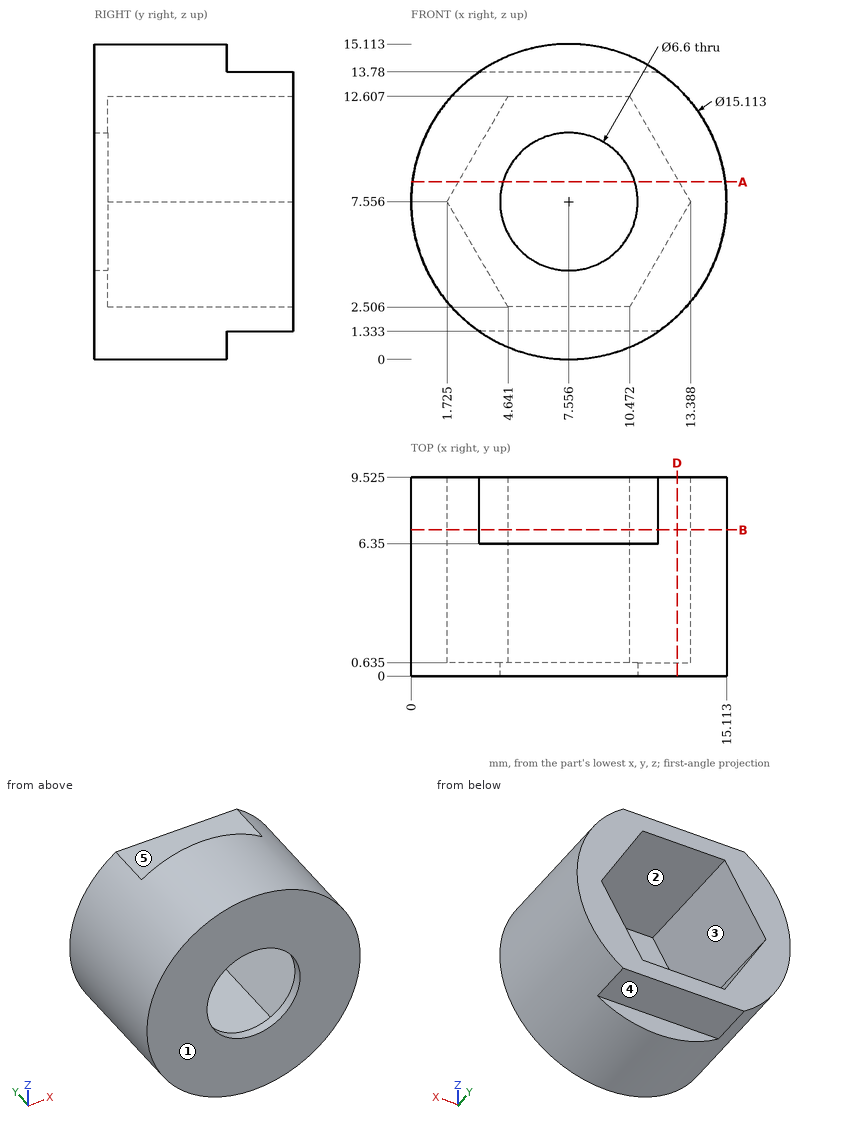
Geometry check sheet. Reference: drawing and pictorial views, mm from the part's lowest x, y, z. A direction names the side the tool comes from. Give positions to 0.01 mm unless a question says otherwise; leave off trailing zeros. Loops run counter-clockwise (first coordinate to the right, second up) from the corner with the lowest first, then second, coordinate; pieces in that order, holes last. Notation, with made-up numbers: (58, 71) -> (73, 71) arc R22 cw to (73, 98) -> close; hole circle Ø6 at (-37.5, 44.25). An arc over 180 degrees is marked (long way). Answer in a Markdown table with one row per item. Add a question column.
1) Material ranges on probe 1 along Z at (x, y) = (8.25, 9.25); probe 2 along Y at (x, z) = (5.5, 11) (1 decimal); probe 3 along Z at (x, y) = (10.5, 8) (1 decimal), recorded low to high. Write a range as from..to.
2) Cross-section at D-D on x = 12.75. Record the boundary of the cut face in (y, z) (1 decimal).
3) Cross-section at B-B on y = 7. Record the boundary of the cut face in (x, z) (1 decimal).
4) Set-up check for the marked faces 1 and 2: record each of +Z, -Z, +X, -X, +Y, -Y from which the full face is reachable in a straight line by a thin tool's end or side.
5) Cross-section at A-A on z = 8.5. Record the boundary of the cut face in (x, y) (1 decimal).
6) Gauge pin test, flat ends, axial feed: P1, Ø1, axis at x = 7, y = 8.5, coming from the -Z side; P2, Ø3.5, axis at x = 6.5, y = 8, coming from the +Z side; P3, Ø2, axis at x = 4, z = 6, coming from the +Y side (1 decimal). Record the tip position at first contact, or that the pin passes through.
7) Draft check along Z on the marked faces 3, 4 and 5. Enter one of: pulls with the +Z half, pulls with the -Z half, needs draft (parallel to the pull), parting line crosses it, or undercut.
Outcome:
| question | item | result |
|---|---|---|
| 1 | probe 1 | z = 1.33..2.51, 12.61..13.78 |
| 1 | probe 2 | y = 0..0.6 |
| 1 | probe 3 | z = 1.3..2.6, 12.6..13.8 |
| 2 | outline | (0, 2.1) -> (9.5, 2.1) -> (9.5, 6.5) -> (0.6, 6.5) -> (0.6, 8.7) -> (9.5, 8.7) -> (9.5, 13) -> (0, 13) -> close |
| 3 | outline | (3.3, 1.3) -> (11.8, 1.3) arc R7.6 ccw to (11.8, 13.8) -> (3.3, 13.8) arc R7.6 ccw to start; hole (1.7, 7.6) -> (4.6, 2.5) -> (10.5, 2.5) -> (13.4, 7.6) -> (10.5, 12.6) -> (4.6, 12.6) -> close |
| 4 | face 1 | +Z, -Z, +X, -X, -Y |
| 4 | face 2 | +Y |
| 5 | outline | (0.1, 0) -> (4.4, 0) -> (4.4, 0.6) -> (2.3, 0.6) -> (2.3, 9.5) -> (0.1, 9.5) -> close; (10.7, 0) -> (15.1, 0) -> (15.1, 9.5) -> (12.8, 9.5) -> (12.8, 0.6) -> (10.7, 0.6) -> close |
| 6 | P1 | stops at z = 1.33 |
| 6 | P2 | stops at z = 15.1 |
| 6 | P3 | stops at y = 0.6 |
| 7 | face 3 | undercut |
| 7 | face 4 | pulls with the -Z half |
| 7 | face 5 | pulls with the +Z half |
